The model under review builds one solid part; all positions refer to its coordinate system, in mm. A direction names the side the tool comes from. Give positions to 0.01 mm unless a question says otherwise; leave off trailing zeros. Order: outer loops, then holes, each group sorted by start corner. A loop starts at its lowest first (then second) coordinate and runs counter-clockwise, first axis right, second up.
```python
from build123d import *

# Parameters (mm, degrees)
SKETCH_1_W          = 25
SKETCH_1_H          = 30
EXTRUDE_1_DEPTH     = 15
SKETCH_2_W          = 21
SKETCH_2_H          = 26
CUT_EXTRUDE_1_DEPTH = 13
SKETCH_3_W          = 21
SKETCH_3_H          = 26
SKETCH_3_W_2        = 18
SKETCH_3_H_2        = 23
EXTRUDE_2_DEPTH     = 3
SKETCH_5_W          = 4.5
SKETCH_5_H          = 6
EXTRUDE_3_DEPTH     = 3
SKETCH_6_R          = 1.6
CUT_EXTRUDE_2_DEPTH = 6
SKETCH_7_W          = 9
SKETCH_7_H          = 8
CUT_EXTRUDE_3_DEPTH = 3


with BuildPart() as part:
    # ｽｹｯﾁ1 → ﾎﾞｽ - 押し出し1 (new body)
    with BuildSketch(Plane.XY):
        with Locations((-71.40312059, 25.678571429)):
            Rectangle(SKETCH_1_W, SKETCH_1_H)
    extrude(amount=EXTRUDE_1_DEPTH)

    # ｽｹｯﾁ2 → ｶｯﾄ - 押し出し1 (cut)
    with BuildSketch(Plane.XY.offset(15)):
        with Locations((-71.40312059, 25.678571429)):
            Rectangle(SKETCH_2_W, SKETCH_2_H)
    extrude(amount=-CUT_EXTRUDE_1_DEPTH, mode=Mode.SUBTRACT)

    # ｽｹｯﾁ3 → ﾎﾞｽ - 押し出し2 (add)
    with BuildSketch(Plane.XY.offset(2)):
        with Locations((-71.40312059, 25.678571429)):
            Rectangle(SKETCH_3_W, SKETCH_3_H)
        with Locations((-71.40312059, 25.678571429)):
            Rectangle(SKETCH_3_W_2, SKETCH_3_H_2, mode=Mode.SUBTRACT)
    extrude(amount=EXTRUDE_2_DEPTH)

    # ｽｹｯﾁ5 → ﾎﾞｽ - 押し出し3 (add)
    with BuildSketch(Plane.XY.offset(2)):
        with Locations((-64.65312059, 19.178571429)):
            Rectangle(SKETCH_5_W, SKETCH_5_H)
        with Locations((-78.15312059, 19.178571429)):
            Rectangle(SKETCH_5_W, SKETCH_5_H)
    extrude(amount=EXTRUDE_3_DEPTH)

    # ｽｹｯﾁ6 → ｶｯﾄ - 押し出し2 (cut, through all)
    with BuildSketch(Plane.XY.offset(5)):
        with Locations((-64.40312059, 19.178571429)):
            Circle(SKETCH_6_R)
        with Locations((-78.40312059, 19.178571429)):
            Circle(SKETCH_6_R)
    extrude(amount=-CUT_EXTRUDE_2_DEPTH, mode=Mode.SUBTRACT)

    # ｽｹｯﾁ7 → ｶｯﾄ - 押し出し3 (cut, through all)
    with BuildSketch(Plane(origin=(0, 12.678571429, 0), x_dir=(1, 0, 0), z_dir=(0, 1, 0))):
        with Locations((-71.40312059, -9)):
            Rectangle(SKETCH_7_W, SKETCH_7_H)
    extrude(amount=-CUT_EXTRUDE_3_DEPTH, mode=Mode.SUBTRACT)


solid = part.part
```
Item 1: Take a section at B-B (z = 13.75). Give the boundary of the cut face in (x, y).
Values found:
outline: (-83.9, 10.68) - (-58.9, 10.68) - (-58.9, 40.68) - (-83.9, 40.68) - close; hole (-81.9, 12.68) - (-60.9, 12.68) - (-60.9, 38.68) - (-81.9, 38.68) - close
Item 2: Take a section at D-D (x = -80.75). Give the boundary of the cut face in (y, z), and give its area (3 significant figures).
Values found:
outline: (10.68, 0) - (40.68, 0) - (40.68, 15) - (38.68, 15) - (38.68, 5) - (12.68, 5) - (12.68, 15) - (10.68, 15) - close
area: 190 mm2
Item 3: For line 1 (X direction, y = 28, z = 4.75); line 2 (Y direction, x = -66.75, z = 12.25); line 3 (X direction, y = 21.5, z = 9.75), list the stretches that pass through material, from the lowest coordinate up.
Values found:
line 1: x = -83.9 to -80.4, -62.4 to -58.9
line 2: y = 10.68 to 12.68, 38.68 to 40.68
line 3: x = -83.9 to -81.9, -60.9 to -58.9
Item 4: Take a section at C-C (y = 15.5). Give the boundary of the cut face in (x, z).
Values found:
outline: (-83.9, 0) - (-58.9, 0) - (-58.9, 15) - (-60.9, 15) - (-60.9, 5) - (-62.4, 5) - (-62.4, 2) - (-80.4, 2) - (-80.4, 5) - (-81.9, 5) - (-81.9, 15) - (-83.9, 15) - close
Item 5: Take a section at A-A (x = -69.75). Give the boundary of the cut face in (y, z), and give its area (3 significant figures).
Values found:
outline: (10.68, 0) - (40.68, 0) - (40.68, 15) - (38.68, 15) - (38.68, 5) - (37.18, 5) - (37.18, 2) - (14.18, 2) - (14.18, 5) - (10.68, 5) - close; (10.68, 13) - (12.68, 13) - (12.68, 15) - (10.68, 15) - close
area: 105 mm2
Item 6: Draft analysis for pull direction Z (two halves, no side actions). For faces 4 (the flat face through (-71, 12, 13)), 5 (the flat face through (-83, 26, 15)), 6 (the flat face through (-75.903, 19, 3)), state which applies: released by +Z, released by -Z, zero draft, split by the parting line, or undercut.
Values found:
face 4: undercut
face 5: released by +Z
face 6: zero draft
Item 7: For faces 1 (the flat face through (-58.903, 25, 7)), 2 (the flat face through (-78, 22.179, 3)), 3 (the flat face through (-75.903, 12, 9)), list the 3-axis set-ups (+Z, -Z, +X, -X, +Y, -Y) from which the entire face can be reached by the end or side of a thin tool; tool diameter is ignored.
Values found:
face 1: +Z, -Z, +X, +Y, -Y
face 2: +Z
face 3: -Y
Item 8: Clearance check with flat-ended pins moving along their axes: pin 1 Ø3 at (x, y) = (-78.4, 19.18) entering from +Z; pin 2 Ø4 at (x, y) = (-77.5, 18.5) entering from +Z. State where each tip first meets the part, or that it passes through.
Values found:
pin 1: passes through
pin 2: stops at z = 5
